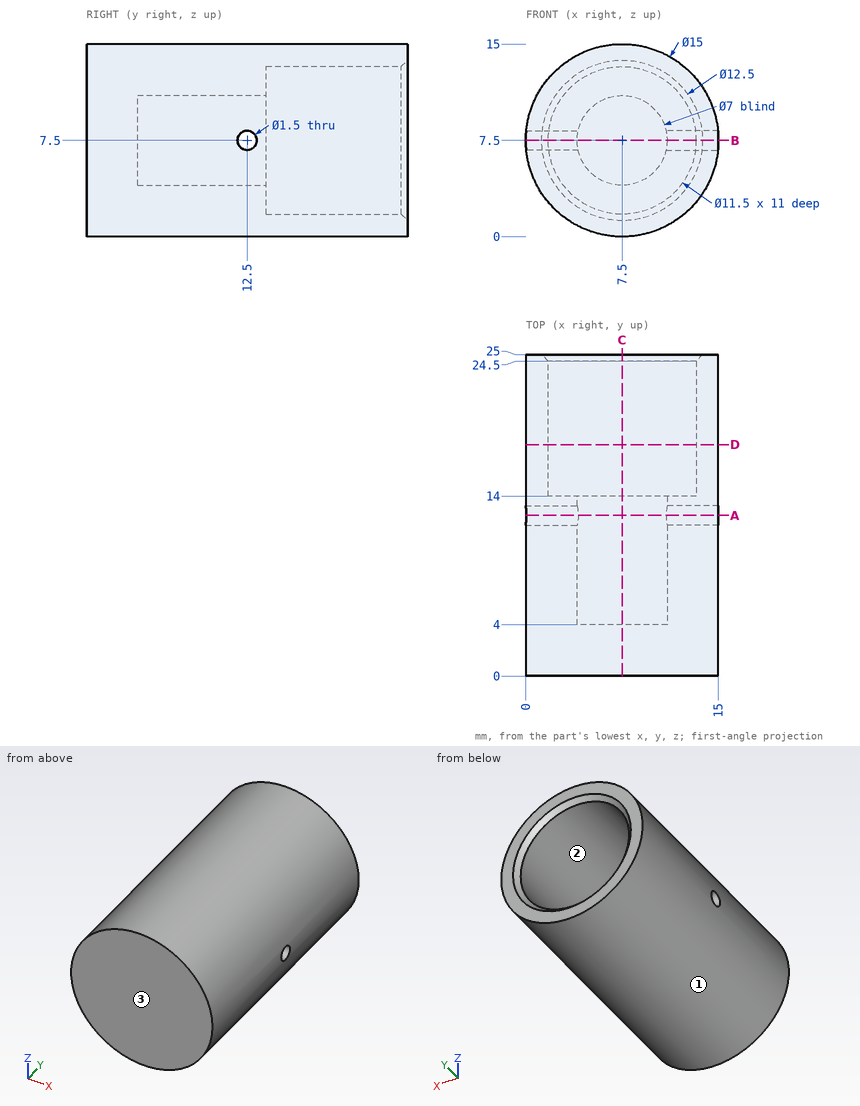
Part print with two shaded views. Sizes in mm from the minimum x, y, z corner. Round coordinates to 2 decimals unless told otherwise and drop trailing zeros. Write each loop counter-clockwise with the first axis right and the second up, starting at its lowest first coordinate (ties: lowest second). Pieces come first, ordered by that corner, then holes. Notation, with made-up numbers: M 47.5,62.5 L 53.5,62.5 A20 ccw 53.5,82.5 Z; hole C 62.25,24 d10. An arc over 180 degrees is marked long. Answer as CSV lines item,"result". Start each with the question number.
1) Mould opens along X. For the marked faces 1, 2 and 3 say: +X half, -X half, draft (parallel to the pull), parting line (faces both ways), or undercut.
2) Drop flat-ended pins along their axis: pin 1 (1.5 mm diameter, centred on y = 12.5, z = 11, fed in from -X); pin 2 (3 mm diameter, centred on x = 9.5, y = 20.5, fed in from -Z); pin 3 (3 mm diameter, centred on y = 13, z = 9.5, fed in from +X). Give the stop position or say it passes through.
3) Band-saw the part on B-B (z = 7.5). List the corners of the cut face in (x, y).
4) Band-saw the part on D-D (y = 18). List the corners of the cut face in (x, z), then the cut area to 3 significant figures.
5) Band-saw the part on C-C (x = 7.5). List the corners of the cut face in (y, z), then the cut area to 3 significant figures.
6) Drill centre lines: L1, parallel to Z at x = 7.5, y = 21.25; L2, parallel to Z at x = 7.5, y = 9.25; L3, parallel to Y at x = 9.5, z = 3. Where is each one in solid material? Low to high.
7) Band-saw the part on A-A (y = 12.5). List the corners of the cut face in (x, z), then the cut area to 3 significant figures.
Worked out:
1,face 1,"parting line"
1,face 2,"undercut"
1,face 3,"draft"
2,pin 1,"x = 0.52"
2,pin 2,"z = 0.02"
2,pin 3,"x = 14.98"
3,outline,"M 0,0 L 15,0 L 15,11.75 L 11,11.75 L 11,4 L 4,4 L 4,11.75 L 0,11.75 Z; M 0,13.25 L 4,13.25 L 4,14 L 1.75,14 L 1.75,24.5 L 1.25,25 L 0,25 Z; M 11,13.25 L 15,13.25 L 15,25 L 13.75,25 L 13.25,24.5 L 13.25,14 L 11,14 Z"
4,outline,"C 7.5,7.5 d15; hole C 7.5,7.5 d11.5"
4,area,"72.8 mm²"
5,outline,"M 0,0 L 25,0 L 25,1.25 L 24.5,1.75 L 14,1.75 L 14,4 L 4,4 L 4,11 L 14,11 L 14,13.25 L 24.5,13.25 L 25,13.75 L 25,15 L 0,15 Z"
5,area,"178 mm²"
6,L1,"0 to 1.75, 13.25 to 15"
6,L2,"0 to 4, 11 to 15"
6,L3,"0 to 14"
7,outline,"M 0.04,6.75 A7.5 ccw 14.96,6.75 L 10.92,6.75 A3.5 cw 4.08,6.75 Z; M 0.04,8.25 L 4.08,8.25 A3.5 cw 10.92,8.25 L 14.96,8.25 A7.5 ccw Z"
7,area,"126 mm²"
